Autodesk Inventor part; units mm, degrees
ref_plane "Work Plane3" through (-63.5, -27, 0) normal (0, 0, -1) x (0, 1, 0)
ref_plane "YZ Plane" through (0, 0, 0) normal (1, 0, 0) x (0, 1, 0)
ref_plane "XZ Plane" through (0, 0, 0) normal (0, 1, 0) x (-1, 0, 0)
ref_plane "Work Plane1" through (0, 0, 0.1) normal (0, 0, 1) x (1, 0, 0)
sketch "Sketch1" plane through (0, 0, 0.1) normal (0, 0, 1) x (1, 0, 0)
  circle A0 centre (-52.5, -39.75) radius 1.5
  circle A1 centre (17.5, -5.25) radius 1.5
  circle A2 centre (-52.5, -5.25) radius 1.5
  circle A3 centre (17.5, -39.75) radius 1.5
  line L0 (-62.5, -18) -> (-24, -18)
  line L1 (-24, -18) -> (-24, -27)
  line L2 (-24, -27) -> (-62.5, -27)
  line L3 (-62.5, -44) -> (-62.5, -27) construction
  line L4 (62.5, -44) -> (-62.5, -44) construction
  line L5 (62.5, -22.5) -> (62.5, -44) construction
  circle A4 centre (43, -22.5) radius 19.5
  line L6 (62.5, -1) -> (62.5, -22.5) construction
  line L7 (-62.5, -1) -> (62.5, -1) construction
  line L8 (-62.5, -18) -> (-62.5, -1) construction
  circle A5 centre (43, -22.5) radius 19.8
  line L9 (23.5, -12.5) -> (-24, -12.5)
  line L10 (23.5, -32.5) -> (-24, -32.5)
  line L11 (23.5, -12.2) -> (-24, -12.2)
  line L12 (23.5, -32.8) -> (-24, -32.8)
  line L13 (-63.5, 0) -> (-63.5, -45)
  line L14 (63.5, 0) -> (-63.5, 0)
  line L15 (-63.5, -45) -> (63.5, -45)
  line L16 (63.5, -45) -> (63.5, 0)
  line L17 (66.6, -48.1) -> (-66.6, -48.1)
  line L18 (-66.6, -48.1) -> (-66.6, 3.1)
  line L19 (-66.6, 3.1) -> (66.6, 3.1)
  line L20 (66.6, 3.1) -> (66.6, -48.1)
  circle A6 centre (17.5, -39.75) radius 1.8
  circle A7 centre (17.5, -5.25) radius 1.8
  circle A8 centre (-52.5, -39.75) radius 1.8
  circle A9 centre (-52.5, -5.25) radius 1.8
  line L21 (23.5, -32.8) -> (26.0899, -32.8)
  line L22 (23.5, -12.2) -> (26.0899, -12.2)
  line L23 (-24, -12.2) -> (-63.5, -12.2)
  line L24 (-24, -32.8) -> (-63.5, -32.8)
  point P0 (0, 0)
  dimension "d0" = 0.3
  dimension "d1" = 0.3
  dimension "d2" = 0.3
  dimension "d3" = 3.1
  dimension "d4" = 0.3
  dimension "d5" = 0.3
  dimension "d6" = 0.3
  dimension "d7" = 0.3
extrude "Extrusion1" add sketch "Sketch1" along normal blind 3 contours A5 L22 L11 L23 L13 L14 L16 L15 L24 L12 L21 | L17 L18 L19 L20
sketch "Sketch2" plane through (0, 0, 0.1) normal (0, 0, -1) x (-1, 0, 0)
  circle A0 centre (52.5, -5.25) radius 1.8 construction
  circle A1 centre (52.5, -39.75) radius 1.8 construction
  circle A2 centre (-17.5, -5.25) radius 1.8 construction
  circle A3 centre (-17.5, -39.75) radius 1.8 construction
  line L0 (-66.6, -48.1) -> (66.6, -48.1)
  line L1 (66.6, -48.1) -> (66.6, 3.1)
  line L2 (66.6, 3.1) -> (-66.6, 3.1)
  line L3 (-66.6, 3.1) -> (-66.6, -48.1)
  line L4 (-26.0899, -12.2) -> (63.5, -12.2) construction
  line L5 (63.5, -12.2) -> (63.5, -32.8) construction
  line L6 (63.5, -32.8) -> (-26.0899, -32.8) construction
  arc A4 (-26.0899, -12.2) -> (-26.0899, -32.8) centre (-43, -22.5) ccw construction
  line L7 (-63.6, 0.1) -> (63.6, 0.1)
  line L8 (63.6, 0.1) -> (63.6, -45.1)
  line L9 (63.6, -45.1) -> (-63.6, -45.1)
  line L10 (-63.6, -45.1) -> (-63.6, 0.1)
  point P0 (0, 0)
  dimension "d10" = 3
extrude "Extrusion2" add sketch "Sketch2" along normal blind 20
sketch "Sketch3" plane through (-66.6, -48.1, 3.1) normal (0, -1, 0) x (1, 0, 0)
  line L0 (3.1, -4.1) -> (130.1, -4.1) construction
  line L1 (3.1, -119.3) -> (3.1, -4.1)
  line L2 (3.1, -119.3) -> (130.1, -119.3)
  line L3 (130.1, -4.1) -> (130.1, -119.3)
  circle A0 centre (122.1, -6.1) radius 1.5 construction
  circle A1 centre (10.1, -6.1) radius 1.5 construction
  circle A2 centre (10.1, -6.1) radius 1.8
  circle A3 centre (122.1, -6.1) radius 1.8
  point P0 (66.6, -3.1)
  dimension "d13" = 0.3
  dimension "d14" = 0.3
extrude "Extrusion3" cut sketch "Sketch3" against normal through all
sketch "Sketch4" plane through (-66.6, -48.1, 3.1) normal (-1, 0, 0) x (0, 0, 1)
  line L0 (-4.1, 3.1) -> (-4.1, 48.1) construction
  line L1 (-4.1, 3.1) -> (-119.3, 3.1) construction
  line L2 (-119.3, 3.1) -> (-119.3, 48.1)
  line L3 (-119.3, 48.1) -> (-4.1, 48.1) construction
  circle A0 centre (-6.1, 9.1) radius 1.5 construction
  circle A1 centre (-6.1, 42.1) radius 1.5 construction
  circle A2 centre (-13, 12) radius 6.65
  line L4 (0, 0) -> (-23, 0)
  line L5 (-23, 0) -> (-23, 51.2)
  line L6 (-23, 25.6) -> (0, 25.6) construction
  line L7 (0, 15.3) -> (0, 35.9)
  circle A3 centre (-13, 39.2) radius 6.65
  point P0 (-3.1, 48.1)
  dimension "d17" = 13.3
  dimension "d18" = 12
  dimension "d19" = 10
extrude "Extrusion4" cut sketch "Sketch4" against normal through all
sketch "Sketch5" plane through (-66.6, -48.1, 3.1) normal (-1, 0, 0) x (0, 0, 1)
  circle A0 centre (-13, 12) radius 6.65
  circle A1 centre (-13, 39.2) radius 6.65
  line L0 (0, 0) -> (-23, 0)
  line L1 (0, 51.2) -> (0, 0)
  line L2 (0, 51.2) -> (-23, 51.2)
  line L3 (-23, 0) -> (-23, 51.2)
  point P0 (-3.1, 48.1)
extrude "Extrusion5" add sketch "Sketch5" along normal blind 6
sketch "Sketch6" plane through (-72.6, -48.1, 3.1) normal (-1, 0, 0) x (0, 0, 1)
  circle A0 centre (-13, 39.2) radius 6.65 construction
  circle A1 centre (-13, 12) radius 6.65 construction
  line L0 (-23, 0) -> (0, 0)
  line L1 (0, 0) -> (0, 51.2)
  line L2 (0, 51.2) -> (-23, 51.2)
  line L3 (-23, 51.2) -> (-23, 0)
  circle A2 centre (-13, 12) radius 4.15
  circle A3 centre (-13, 39.2) radius 4.15
  point P0 (-3.1, 48.1)
  dimension "d24" = 8.3
  dimension "d25" = 8.3
extrude "Extrusion6" add sketch "Sketch6" along normal blind 3
ref_plane "Work Plane2" through (0, -45.1, 0.1) normal (1, 0, 0) x (0, 0, -1)
mirror "Mirror1" about plane through (0, -45.1, 0.1) normal (1, 0, 0) of "Extrusion5", "Extrusion6"
ref_plane "Work Plane3" through (-63.5, -27, 0) normal (0, 0, -1) x (0, 1, 0)
sketch "Sketch7" plane through (0, 0, 3.1) normal (0, 0, 1) x (1, 0, 0)
  circle A0 centre (-52.5, -5.25) radius 1.8
  circle A1 centre (-52.5, -39.75) radius 1.8
  circle A2 centre (17.5, -5.25) radius 1.8
  circle A3 centre (17.5, -39.75) radius 1.8
  line L0 (75.6, -48.1) -> (-75.6, -48.1)
  line L1 (75.6, -48.1) -> (75.6, 3.1)
  line L2 (-75.6, 3.1) -> (75.6, 3.1)
  line L3 (-75.6, -48.1) -> (-75.6, 3.1)
  line L4 (26.0899, -32.8) -> (-63.5, -32.8)
  line L5 (-63.5, -32.8) -> (-63.5, -12.2)
  line L6 (-63.5, -12.2) -> (26.0899, -12.2)
  arc A4 (26.0899, -32.8) -> (26.0899, -12.2) centre (43, -22.5) ccw
  line L7 (-63.5, -12.2) -> (-63.5, -32.8)
  line L8 (-63.6, 0.1) -> (-63.6, -45.1) construction
  arc A5 (-63.5, -12.2) -> (-63.5, -32.8) centre (24.6083, -22.5) ccw
  point P0 (0, 0)
  point P1 (-63.6, -22.5)
  point P2 (-64.1, -22.5)
  dimension "d28" = 0.5
extrude "Extrusion7" cut sketch "Sketch7" against normal blind 5 contours A5 L5
properties part number "Syringe Pump Holder"
Could you check a few things on this model? Use its own coordinates, in mm. A direction names the side the tool comes from. Coordinates: 2 decimals unless noted, no trailing zeros. Order: outer loops, then holes, each group sorted by start corner. A loop starts at its lowest first (then second) coordinate and runs counter-clockwise, first axis right, second up. Notation, with made-up numbers: (45.5, -9.75) - (52.5, -9.75) arc R26 cw to (52.5, 25.25) - close; hole circle Ø6 at (44.25, 62.5). An arc over 180 degrees is marked (long way). Answer in a Markdown table with one row per item. Add a question column.
(1) If we mould it in two halves opening along Y, with no side actions, what happens to faces 6 (the face through (-74.08, -4.85, -10.8)), 7 (the face through (-1, 3.1, -9)), 8 (the face through (-75.6, -22, -9))? For each: released by +Y, released by -Y, zero draft, split by the parting line, or undercut.
(2) Will these pins go through, and if not, where does the flat tip stop? pin 1 (10.5 mm diameter, centred on y = -10.5, z = -8.5, fed in from -X); pin 2 (4 mm diameter, centred on x = -2, y = -33, fed in from -Z).
(3) If we section it at B-B, the plane y = -22.5: Please give me the cut outline in (x, z).
(4) On a 3-axis mill with a long thin cutter (end or side, diameter ignored), from which of +Z, -Z, +X, -X, +Y, -Y can I reach the whole of each face in a straight line? I mean faces 1 (the face through (-64.1, -22.4, 0.6)), 2 (the face through (-19, -32.8, 2)), 3 (the face through (-56.734, 1.579, -1.215)), 4 (the face through (1, 0.1, -10)), 5 (the face through (72.6, -33, -13)). Say none if no direction works.
(5) I need wall thicknesses on L1, parallel to Y at x = -74.4, z = -9.9; L2, parallel to X at y = -41, z = -10.5; L3, parallel to Y at x = 22, z = -2.25. Which ranges of each line are inside material? Lowest first, please.
(6) If we section it at A-A, the plane x = -52.5: Please give me the cut outline in (y, z).
(7) If we section it at C-C, the plane x = 65: Please give me the cut outline in (y, z), then the cut area to 3 significant figures.
(8) If we section it at D-D, the plane x = -27.5: Please give me the cut outline in (y, z).
Results are:
| question | item | result |
|---|---|---|
| 1 | face 6 | undercut |
| 1 | face 7 | released by +Y |
| 1 | face 8 | zero draft |
| 2 | pin 1 | stops at x = -75.6 |
| 2 | pin 2 | stops at z = 0.1 |
| 3 | outline | (-75.6, -19.9) - (-63.6, -19.9) - (-63.6, -1.9) - (-64.1, -1.9) - (-64.1, 3.1) - (-75.6, 3.1) - close; (62.8, 0.1) - (63.6, 0.1) - (63.6, -19.9) - (75.6, -19.9) - (75.6, 3.1) - (62.8, 3.1) - close |
| 4 | face 1 | +Z |
| 4 | face 2 | +Z, -Z |
| 4 | face 3 | +Y, -Y |
| 4 | face 4 | -Z |
| 4 | face 5 | none |
| 5 | L1 | y = -48.1 to -40.25, -31.95 to -13.05, -4.75 to 3.1 |
| 5 | L2 | x = -75.6 to -72.6, 72.6 to 75.6 |
| 5 | L3 | y = -48.1 to -45.1, 0.1 to 3.1 |
| 6 | outline | (-48.1, -19.9) - (-45.1, -19.9) - (-45.1, 0.1) - (-41.55, 0.1) - (-41.55, 3.1) - (-48.1, 3.1) - close; (-37.95, 0.1) - (-32.8, 0.1) - (-32.8, 3.1) - (-37.95, 3.1) - close; (-12.2, 0.1) - (-7.05, 0.1) - (-7.05, 3.1) - (-12.2, 3.1) - close; (-3.45, 0.1) - (0.1, 0.1) - (0.1, -19.9) - (3.1, -19.9) - (3.1, 3.1) - (-3.45, 3.1) - close |
| 7 | outline | (-48.1, -19.9) - (3.1, -19.9) - (3.1, 3.1) - (-48.1, 3.1) - close; hole circle Ø13.3 at (-36.1, -9.9); hole circle Ø13.3 at (-8.9, -9.9) |
| 7 | area | 900 mm2 |
| 8 | outline | (-48.1, -19.9) - (-45.1, -19.9) - (-45.1, 0.1) - (-32.8, 0.1) - (-32.8, 3.1) - (-48.1, 3.1) - close; (-12.2, 0.1) - (0.1, 0.1) - (0.1, -19.9) - (3.1, -19.9) - (3.1, 3.1) - (-12.2, 3.1) - close |
